Input: part model. Units: mm. Frame: model coordinates. Face numbers are marked on the shaded views. A direction names the side the tool comes from. Round coordinates to 2 decimals unless told otherwise and drop trailing zeros. Loops run counter-clockwise (first coordinate to the right, second up) from the corner with the lowest first, then second, coordinate; pieces in that order, holes last. Notation, with made-up numbers: (-23, 63) -> (-17, 63) arc R23 cw to (-17, 88) -> close; hole circle Ø11 at (51.25, 89). An arc over 180 degrees is marked (long way). Answer in a Markdown table with one row per item. Add a question column.
Q1. Pin query (flat end, axial travel): pin 1 (6.5 mm diameter, centred on x = 6, y = -1, fed in from -Z) (3 decimals); pin 2 (3 mm diameter, centred on x = 9, z = -5.5, fed in from +Y); pin 3 (2.5 mm diameter, centred on x = 8.5, z = 1, fed in from -Y); pin 4 (2.5 mm diameter, centred on y = -5.87, z = -4.85, fed in from -X). Return the tip coordinate at first contact, or that it passes through.
Q2. Ray query, L1, parallel to Z at x = 8.5, y = -6; L2, parallel to Y at x = 3.5, z = -4.75; L3, parallel to Z at x = 9, y = -9.5. Return the intervals inside material, ascending. Write a range as from..to.
Q3. Mould query, pull axis Z, two halves, no side actions, for the marked faces 4, 5, 6 and 7. Classes: pulls with the +Z half, pulls with the -Z half, needs draft (parallel to the pull), parting line crosses it, or undercut.
Q4. Section A-A, the plane x = 6.5. Output: boundary loops of the cut face in (y, z), and give its area (3 significant figures).
Q5. Section D-D, the plane z = 1. Output: boundary loops of the cut face in (x, y), and give its area (3 significant figures).
Q6. Section B-B, the plane z = -3.75. Output: boundary loops of the cut face in (x, y).
Q7. Reachability of the marked faces 1, 2 and 3 from +Z, -Z, +X, -X, +Y, -Y: full face, straight path, thin tool, end or side. Return the list, or none.
Q8. Section C-C, the plane y = 1. Output: boundary loops of the cut face in (x, z).
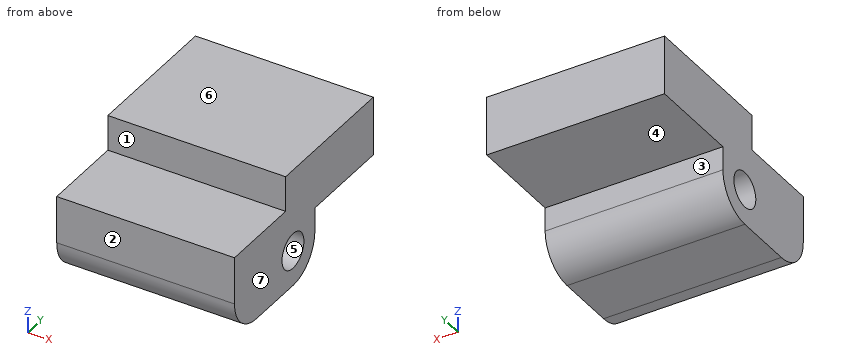
```python
from build123d import *

# Parameters (mm, degrees)
SKETCH1_R           = 1.5
BOSS_EXTRUDE1_DEPTH = 15


with BuildPart() as part:
    # Sketch1 → Boss-Extrude1 (new body)
    with BuildSketch(Plane(origin=(0, 0, 0), x_dir=(0, 0, -1), z_dir=(1, 0, 0))):
        with BuildLine():
            Line((-2.147887324, 5.126760563), (2.852112676, 5.126760563))
            Line((2.852112676, 5.126760563), (2.852112676, -2.873239437))
            Line((2.852112676, -2.873239437), (4.852112676, -2.873239437))
            ThreePointArc((4.852112676, -2.873239437), (6.97343302, -3.751919093), (7.852112676, -5.873239437))
            Line((7.852112676, -5.873239437), (7.852112676, -10.873239437))
            ThreePointArc((7.852112676, -10.873239437), (6.97343302, -12.99455978), (4.852112676, -13.873239437))
            Line((4.852112676, -13.873239437), (0.852112676, -13.873239437))
            Line((0.852112676, -13.873239437), (0.852112676, -6.873239437))
            Line((0.852112676, -6.873239437), (-2.147887324, -6.873239437))
            Line((-2.147887324, -6.873239437), (-2.147887324, 5.126760563))
        make_face()
        with Locations((4.852112676, -5.873239437)):
            Circle(SKETCH1_R, mode=Mode.SUBTRACT)
    extrude(amount=BOSS_EXTRUDE1_DEPTH)


solid = part.part
```
Answer block:
| question | item | result |
|---|---|---|
| 1 | pin 1 | z = -7.375 |
| 1 | pin 2 | y = -2.87 |
| 1 | pin 3 | y = -6.87 |
| 1 | pin 4 | through |
| 2 | L1 | -7.85..-6.35, -3.36..2.15 |
| 2 | L2 | -13.87..-7.37, -4.38..-2.87 |
| 2 | L3 | -7.85..-0.85 |
| 3 | face 4 | pulls with the -Z half |
| 3 | face 5 | undercut |
| 3 | face 6 | pulls with the +Z half |
| 3 | face 7 | needs draft |
| 4 | outline | (-13.87, -4.85) arc R3 ccw to (-10.87, -7.85) -> (-5.87, -7.85) arc R3 ccw to (-2.87, -4.85) -> (-2.87, -2.85) -> (5.13, -2.85) -> (5.13, 2.15) -> (-6.87, 2.15) -> (-6.87, -0.85) -> (-13.87, -0.85) -> close; hole circle Ø3 at (-5.87, -4.85) |
| 4 | area | 118 mm^2 |
| 5 | outline | (0, -6.87) -> (15, -6.87) -> (15, 5.13) -> (0, 5.13) -> close |
| 5 | area | 180 mm^2 |
| 6 | outline | (0, -13.87) -> (15, -13.87) -> (15, -6.89) -> (0, -6.89) -> close; (0, -4.86) -> (15, -4.86) -> (15, -2.87) -> (0, -2.87) -> close |
| 7 | face 1 | +Z, +X, -X, -Y |
| 7 | face 2 | +Z, -Z, +X, -X, -Y |
| 7 | face 3 | -Z, +X, -X, +Y |
| 8 | outline | (0, -2.85) -> (15, -2.85) -> (15, 2.15) -> (0, 2.15) -> close |
